Part model, mm, in its own coordinate system. Give positions to 0.01 mm unless a question says otherwise; leave off trailing zeros. Write each loop counter-clockwise with the first axis right and the second up, starting at its lowest first coordinate (ties: lowest second). Pieces come first, ordered by that corner, then holes.
from build123d import *

# Parameters (mm, degrees)
SKETCH_1_R               = 19
SKETCH_1_R_2             = 17
EXTRUDE_1_DEPTH          = 300
CUT_EXTRUDE_1_DEPTH      = 20
PATTERN_CIRCULAR_1_COUNT = 4


with BuildPart() as part:
    # 草图1 → 拉伸-薄壁1 (new body)
    with BuildSketch(Plane(origin=(0, 0, 0), x_dir=(1, 0, 0), z_dir=(0, 1, 0))):
        Circle(SKETCH_1_R)
        Circle(SKETCH_1_R_2, mode=Mode.SUBTRACT)
    extrude(amount=EXTRUDE_1_DEPTH)

    # 草图3 → 切除-拉伸1 (cut)
    with BuildSketch(Plane(origin=(0, 300, 0), x_dir=(1, 0, 0), z_dir=(0, 1, 0))):
        Polygon((0, 0), (0, 19), (2, 19), align=None)
    cut_extrude_1 = extrude(amount=-CUT_EXTRUDE_1_DEPTH, mode=Mode.SUBTRACT)

    # 阵列(圆周)1: 切除-拉伸1 ×4 about axis
    pattern_circular_1_axis = Axis((0, 300, 0), (0, -1, 0))
    for i in range(1, PATTERN_CIRCULAR_1_COUNT):
        add(cut_extrude_1.rotate(pattern_circular_1_axis, i * 360 / PATTERN_CIRCULAR_1_COUNT), mode=Mode.SUBTRACT)


solid = part.part
1) Saw through at B-B (x = -7). Write the cut outline in (y, z).
Check result:
outline: (0, -17.66) - (300, -17.66) - (300, -15.49) - (0, -15.49) - close; (0, 15.49) - (300, 15.49) - (300, 17.66) - (0, 17.66) - close
2) Saw through at C-C (y = 68). Write the cut outline in (x, z), and give its area (3 significant figures).
Check result:
outline: circle Ø38 at (0, 0); hole circle Ø34 at (0, 0)
area: 226 mm2
3) Mould opens along Z. For faces 1 (the flat face through (-13, 300, 12)), 2 (the cylindrical face through (17.55, 147.9, 7.28)), 3 (the cylindrical face through (16.215, 147.9, -5.106)) say: +Z half, -Z half, draft (parallel to the pull), parting line (faces both ways), or undercut.
Check result:
face 1: draft
face 2: parting line
face 3: undercut
4) Saw through at A-A (z = -12). Write the cut outline in (x, y), and give its area (3 significant figures).
Check result:
outline: (-14.73, 0) - (-12.04, 0) - (-12.04, 300) - (-14.73, 300) - close; (12.04, 0) - (14.73, 0) - (14.73, 300) - (12.04, 300) - close
area: 1,610 mm2
5) Flat gauge pins, fed straight in: P1, Ø1, axis at x = -17.5, y = 292, coming from the -Z side; P2, Ø5, axis at x = -5.5, y = 177.5, coming from the +Z side; P3, Ø8, axis at x = 8.5, y = 156.5, coming from the -Z side; P4, Ø12, axis at x = -9, z = -2, coming from the +Y side. Where does each tip first touch, or does it go through?
Check result:
P1: stops at z = -8.49
P2: stops at z = 18.76
P3: stops at z = -18.46
P4: passes through
6) Drill centre lines: L1, parallel to X at y = 158, z = 0; L2, parallel to Z at x = 12.5, y = 190. Where is each one in solid material? Low to high.
Check result:
L1: x = -19 to -17, 17 to 19
L2: z = -14.31 to -11.52, 11.52 to 14.31
